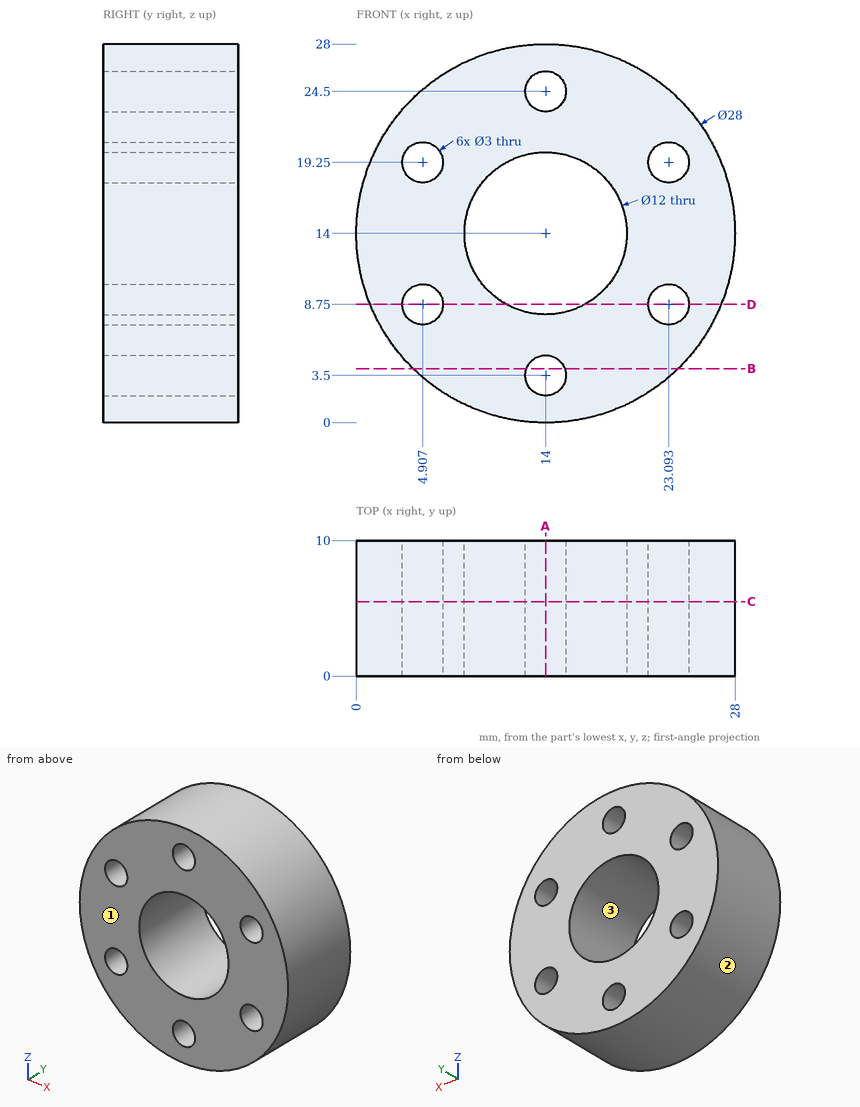
Verification items for this drawing (mm, ordinates from the low corner). Coordinates: 2 decimals unless noted, no trailing zeros. Order: outer loops, then holes, each group sorted by start corner. A loop starts at its lowest first (then second) coordinate and runs counter-clockwise, first axis right, second up.
Q1. Thickness scan on probe 1 along Z at (x, y) = (14, 6); probe 2 along Z at (x, y) = (13.25, 3); probe 3 along X at (y, z) = (6.25, 19.25) (1 decimal). Record the ranges inside material, lowest first.
Reply:
probe 1: z = 0 to 2, 5 to 8, 20 to 23, 26 to 28
probe 2: z = 0.02 to 2.2, 4.8 to 8.05, 19.95 to 23.2, 25.8 to 27.98
probe 3: x = 1 to 3.4, 6.4 to 11.1, 16.9 to 21.6, 24.6 to 27
Q2. Depth check by flat-ended pin: pin 1 Ø1 at (x, y) = (12.5, 9) entering from -Z. Enter the tip coordinate at first touch or a pass-through.
Reply:
pin 1: stops at z = 0.04
Q3. Sectioned sample at A-A on x = 14. Record the cut outline in (y, z), and give its area (3 significant figures).
Reply:
outline: (0, 0) - (10, 0) - (10, 2) - (0, 2) - close; (0, 5) - (10, 5) - (10, 8) - (0, 8) - close; (0, 20) - (10, 20) - (10, 23) - (0, 23) - close; (0, 26) - (10, 26) - (10, 28) - (0, 28) - close
area: 100 mm2
Q4. Sectioned sample at B-B on z = 4. Record the cut outline in (x, y).
Reply:
outline: (4.2, 0) - (12.59, 0) - (12.59, 10) - (4.2, 10) - close; (15.41, 0) - (23.8, 0) - (23.8, 10) - (15.41, 10) - close
Q5. Sectioned sample at D-D on z = 8.75. Record the cut outline in (x, y) (1 decimal).
Reply:
outline: (1, 0) - (3.4, 0) - (3.4, 10) - (1, 10) - close; (6.4, 0) - (11.1, 0) - (11.1, 10) - (6.4, 10) - close; (16.9, 0) - (21.6, 0) - (21.6, 10) - (16.9, 10) - close; (24.6, 0) - (27, 0) - (27, 10) - (24.6, 10) - close
Q6. Draft check along X on the marked faces 1, 2 and 3. Enter one of: released by +X, released by -X, zero draft, split by the parting line, or undercut.
Reply:
face 1: zero draft
face 2: split by the parting line
face 3: undercut
Q7. Sectioned sample at C-C on y = 5.5. Record the cut outline in (x, z).
Reply:
outline: circle Ø28 at (14, 14); hole circle Ø3 at (4.91, 8.75); hole circle Ø3 at (4.91, 19.25); hole circle Ø12 at (14, 14); hole circle Ø3 at (14, 3.5); hole circle Ø3 at (14, 24.5); hole circle Ø3 at (23.09, 8.75); hole circle Ø3 at (23.09, 19.25)
